CAD build for the part. Positions are in the model's coordinates, mm. A direction names the side the tool comes from. Round coordinates to 2 decimals unless told otherwise and drop trailing zeros. Order: outer loops, then holes, each group sorted by start corner. A loop starts at its lowest first (then second) coordinate and runs counter-clockwise, first axis right, second up. Notation, with made-up numbers: M 0.5,1 L 34.5,1 A27 cw 34.5,24 Z; hole C 11.25,65.5 d6. An arc over 180 degrees is marked long. Answer as a JSON object with one key per item and string values.
```python
from build123d import *

# Parameters (mm, degrees)
BOSS_EXTRUDE2_DEPTH = 20
BOSS_EXTRUDE3_DEPTH = 10


with BuildPart() as part:
    # Sketch1 → Boss-Extrude2 (new body)
    with BuildSketch(Plane.XY):
        with BuildLine():
            Line((50, 35), (-40, 35))
            ThreePointArc((-40, 35), (5, 57.290269493), (50, 35))
        make_face()
    extrude(amount=-BOSS_EXTRUDE2_DEPTH)

    # Sketch3 → Boss-Extrude3 (add)
    with BuildSketch(Plane.XY):
        with BuildLine():
            Line((-23.995294076, 49.29407429), (-9.782013153, 55.324768004))
            ThreePointArc((-9.782013153, 55.324768004), (-19.193781446, 57.742200687), (-23.995294076, 49.29407429))
        make_face()
        with BuildLine():
            Line((19.274375244, 55.45966824), (33.55614581, 49.553545892))
            ThreePointArc((33.55614581, 49.553545892), (28.681224063, 57.986001061), (19.274375244, 55.45966824))
        make_face()
    extrude(amount=-BOSS_EXTRUDE3_DEPTH)


solid = part.part
```
Item 1: Saw through at C-C on z = -15.5. List the corners of the cut face in (x, y).
Worked answers:
{"outline": "M -40,35 L 50,35 A56.57 ccw Z"}
Item 2: Saw through at A-A on y = 56.5. List the corners of the cut face in (x, z).
Worked answers:
{"outline": "M -21.22,-10 L -10.92,-10 L -10.92,0 L -21.22,0 Z; M -4.42,-20 L 14.42,-20 L 14.42,0 L -4.42,0 Z; M 20.23,-10 L 31.02,-10 L 31.02,0 L 20.23,0 Z"}
Item 3: Saw through at B-B on y = 51.5. List the corners of the cut face in (x, z).
Worked answers:
{"outline": "M -23.99,-10 L -19.93,-10 L -19.93,-20 L 29.93,-20 L 29.93,-10 L 33.57,-10 L 33.57,0 L -23.99,0 Z"}
Item 4: 3-axis set-ups, long thin cutter, end or side, ignore diameter. For faces 1 (the flat face through (6, 44, -20)), 2 (the flat face through (-19, 55, -10)): which of +Z, -Z, +X, -X, +Y, -Y reach the whole face in a straight line?
Worked answers:
{"face 1": "-Z, +X, -X, +Y, -Y", "face 2": "-Z, -X, +Y"}
Item 5: Drop flat-ended pins along their axis: pin 1 Ø1 at (x, z) = (30, -14) entering from +Y; pin 2 Ø1 at (x, y) = (-22, 56) entering from -Z; pin 3 Ø10 at (y, z) = (47, -15) entering from -X. Give the stop position or say it passes through.
Worked answers:
{"pin 1": "stops at y = 51.71", "pin 2": "stops at z = -10", "pin 3": "stops at x = -33.68"}
Item 6: Wall check: line 1 along Z through (x, y) = (25.5, 54.5); line 2 along X through (y, z) = (42.75, -11); line 3 along Y through (x, z) = (12, -14.5). Give the ranges that are in metal, low to high. Write a range as [from, to].
Worked answers:
{"line 1": "z = [-10, 0]", "line 2": "x = [-32.86, 42.86]", "line 3": "y = [35, 56.86]"}
Item 7: Saw through at D-D on x = 12. List the corners of the cut face in (y, z).
Worked answers:
{"outline": "M 35,-20 L 56.86,-20 L 56.86,0 L 35,0 Z"}
Item 8: Two-plate mould, pull along X, no slides. Class faces 3 (the cylindrical face through (4.272, 57.286, -9.86)), 4 (the cylindrical face through (-19.059, 57.798, -4.93)), 5 (the flat face through (6, 44, 0)): released by +X, released by -X, zero draft, split by the parting line, or undercut.
Worked answers:
{"face 3": "undercut", "face 4": "undercut", "face 5": "zero draft"}
